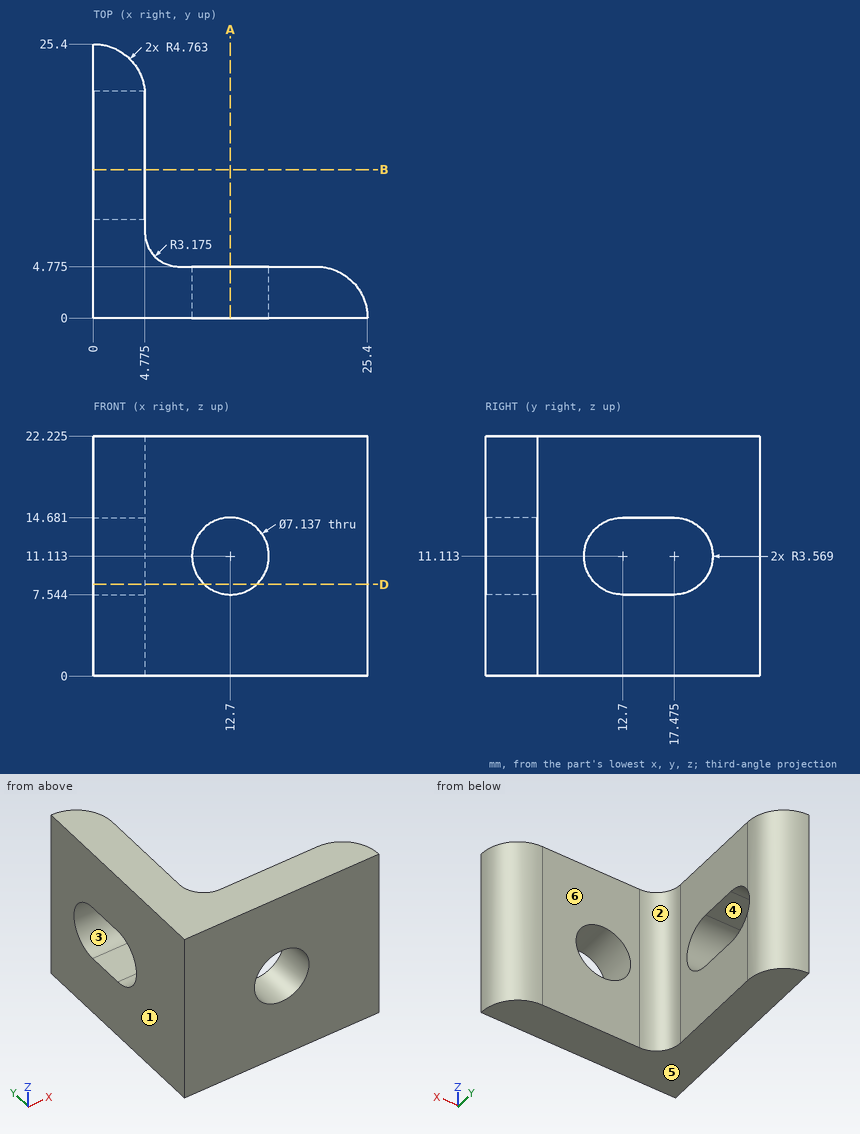
Study the drawing (mm; zero at the part's minimum x, y, z) and answer. A direction names the side the tool comes from. Give positions to 0.01 mm unless a question says otherwise; leave off trailing zeros. Write each loop counter-clockwise with the first axis right and the second up, starting at its lowest first coordinate (ties: lowest second). Pieces come first, ordered by that corner, then holes. Notation, with made-up numbers: (53, 27) - (97, 27) arc R14 ccw to (97, 33) - close; hole circle Ø10 at (24, 56.5). An arc over 180 degrees is marked (long way). Use a Markdown table: item, result.
1. Section D-D on z = 8.5 is taken. Count the separate pieces of the cut face and the enclosed holes in it, plus the area to 3 significant figures.
Values follow:
| item | result |
|---|---|
| separate pieces | 3 |
| enclosed holes | 0 |
| area | 143 mm² |
2. For a pull along Y with two mould halves and no side action, classify the marked faces 1, 2 and 3 as released by +Y, released by -Y, zero draft, split by the parting line, or undercut.
Values follow:
| item | result |
|---|---|
| face 1 | zero draft |
| face 2 | released by +Y |
| face 3 | undercut |
3. A tool of negligible diameter and unlimited length cuts with its end or side. For the marked faces 4, 5 and 6, from which of +Z, -Z, +X, -X, +Y, -Y can it reach the whole face along a straight path? Write none if from no direction.
Values follow:
| item | result |
|---|---|
| face 4 | +X, -X |
| face 5 | -Z, +X, -X, +Y, -Y |
| face 6 | +Z, -Z, +X, +Y |
4. Section A-A on x = 12.7 is taken. Write down the section's boundary in (y, z) (1 decimal).
Values follow:
| item | result |
|---|---|
| outline | (0, 0) - (4.8, 0) - (4.8, 7.5) - (0, 7.5) - close; (0, 14.7) - (4.8, 14.7) - (4.8, 22.2) - (0, 22.2) - close |
5. Find the intervals of material crossed by probe 1 along Z at (x, y) = (12.7, 1.1) (1 decimal); probe 2 along X at (y, z) = (1.25, 12) (1 decimal); probe 3 along Z at (x, y) = (4.25, 9.75) (1 decimal), in increasing order. Write a range as from..to.
Values follow:
| item | result |
|---|---|
| probe 1 | z = 0..7.5, 14.7..22.2 |
| probe 2 | x = 0..9.2, 16.2..25.2 |
| probe 3 | z = 0..9.1, 13.1..22.2 |
6. Each of these flat-tipped pins is pushed along its axis until it touches: P1, Ø4, axis at y = 15, z = 6, coming from the +X side (1 decimal); P2, Ø4, axis at y = 4.5, z = 8, coming from the +X side; P3, Ø1, axis at x = 3.5, z = 16.5, coming from the +Y side (1 decimal). Where does it stop, or does it pass through?
Values follow:
| item | result |
|---|---|
| P1 | stops at x = 4.8 |
| P2 | stops at x = 24.7 |
| P3 | stops at y = 24.3 |
